```python
from build123d import *

# Parameters (mm, degrees)
BOSS_EXTRU_1_DEPTH      = 3
CONG_1_R                = 5
ESQUISSE2_R             = 1
ENL_V_MAT_EXTRU_1_DEPTH = 257.837010573
D_GAGEMENT_M31_D        = 3.4
ESQUISSE5_R             = 12
ESQUISSE5_R_2           = 11
ESQUISSE5_R_3           = 1.5
ESQUISSE5_R_4           = 1
ESQUISSE5_W             = 50
ESQUISSE5_H             = 10
ENL_V_MAT_EXTRU_2_DEPTH = 257.837010573
D_GAGEMENT_M32_D        = 3.4
D_GAGEMENT_M32_DEPTH    = 3


with BuildPart() as part:
    # Esquisse1 → Boss.-Extru.1 (new body)
    with BuildSketch(Plane(origin=(0, 0, 0), x_dir=(1, 0, 0), z_dir=(0, 1, 0))):
        Polygon((-92.5, 0), (92.5, 0), (132.5, 40), (132.5, 220), (102.5, 220), (85.179491924, 190), (-85.179491924, 190), (-102.5, 220), (-132.5, 220), (-132.5, 40), align=None)
    extrude(amount=BOSS_EXTRU_1_DEPTH)

    # Congé1
    cong_1_edges = [part.edges().sort_by_distance(p)[0] for p in [
        (92.5, 1.5, 0),
        (-92.5, 1.5, 0),
        (-132.5, 1.5, -40),
        (-132.5, 1.5, -220),
        (-102.5, 1.5, -220),
        (-85.179491924, 1.5, -190),
        (85.179491924, 1.5, -190),
        (102.5, 1.5, -220),
        (132.5, 1.5, -220),
        (132.5, 1.5, -40),
    ]]
    fillet(cong_1_edges, radius=CONG_1_R)

    # Esquisse2 → Enlèv. mat.-Extru.1 (cut, through all)
    with BuildSketch(Plane.XZ):
        with Locations(Location((-70, -8, 0), (0, 0, 270))):
            Circle(ESQUISSE2_R)
        with Locations(Location((-124.5, -70, 0), (0, 0, 270))):
            Circle(ESQUISSE2_R)
        with Locations(Location((-124.5, -212, 0), (0, 0, 270))):
            Circle(ESQUISSE2_R)
        with Locations(Location((124.5, -212, 0), (0, 0, 90))):
            Circle(ESQUISSE2_R)
        with Locations(Location((124.5, -70, 0), (0, 0, 90))):
            Circle(ESQUISSE2_R)
        with Locations(Location((70, -8, 0), (0, 0, 90))):
            Circle(ESQUISSE2_R)
    extrude(amount=-ENL_V_MAT_EXTRU_1_DEPTH, mode=Mode.SUBTRACT)

    # Dégagement M31 (through all)
    with Locations(Plane(origin=(0, 0, 0), x_dir=(-1, 0, 0), z_dir=(0, -1, 0))):
        with Locations((-70, 8), (-124.5, 70), (-124.5, 212), (124.5, 212), (124.5, 70), (70, 8)):
            Hole(D_GAGEMENT_M31_D / 2)

    # Esquisse5 → Enlèv. mat.-Extru.2 (cut, through all)
    with BuildSketch(Plane.XZ):
        with Locations(Location((-97.5, -36, 0), (0, 0, 270))):
            Circle(ESQUISSE5_R)
        with Locations(Location((97.5, -55, 0), (0, 0, 270))):
            Circle(ESQUISSE5_R_2)
        with Locations(Location((97.5, -86, 0), (0, 0, 270))):
            Circle(ESQUISSE5_R_3)
        with Locations(Location((97.5, -24, 0), (0, 0, 270))):
            Circle(ESQUISSE5_R_3)
        with Locations(Location((-35, -138, 0), (0, 0, 270))):
            Circle(ESQUISSE5_R_4)
        with Locations(Location((-35, -82, 0), (0, 0, 270))):
            Circle(ESQUISSE5_R_4)
        with Locations(Location((35, -130, 0), (0, 0, 270))):
            Circle(ESQUISSE5_R_4)
        with Locations(Location((35, -90, 0), (0, 0, 270))):
            Circle(ESQUISSE5_R_4)
        with Locations(Location((0, -166, 0), (0, 0, 270))):
            Circle(ESQUISSE5_R_3)
        with Locations(Location((-54.5, -54, 0), (0, 0, 270))):
            Circle(ESQUISSE5_R_3)
        with Locations(Location((54.5, -54, 0), (0, 0, 270))):
            Circle(ESQUISSE5_R_3)
        with Locations(Location((-87.5, -74, 0), (0, 0, 270))):
            Circle(ESQUISSE5_R_3)
        with Locations(Location((-87.5, -165, 0), (0, 0, 270))):
            Circle(ESQUISSE5_R_3)
        with Locations(Location((-32.335, -50, 0), (0, 0, 270))):
            Circle(ESQUISSE5_R_3)
        with Locations(Location((-32.335, -10, 0), (0, 0, 270))):
            Circle(ESQUISSE5_R_3)
        with Locations(Location((32.335, -10, 0), (0, 0, 270))):
            Circle(ESQUISSE5_R_3)
        with Locations(Location((32.335, -50, 0), (0, 0, 270))):
            Circle(ESQUISSE5_R_3)
        with Locations((2.5, -82)):
            Rectangle(ESQUISSE5_W, ESQUISSE5_H)
    extrude(amount=-ENL_V_MAT_EXTRU_2_DEPTH, mode=Mode.SUBTRACT)

    # Dégagement M32
    with Locations(Plane(origin=(0, 3, 0), x_dir=(1, 0, 0), z_dir=(0, 1, 0))):
        with Locations((97.5, 86), (97.5, 24), (-54.5, 54), (54.5, 54), (0, 166), (-87.5, 74), (-87.5, 165), (-32.335, 50), (-32.335, 10), (32.335, 10), (32.335, 50), (-35, 138), (-35, 82), (35, 90), (35, 130)):
            Hole(D_GAGEMENT_M32_D / 2, depth=D_GAGEMENT_M32_DEPTH)


solid = part.part
```
Could you check a few things on this model? Use its own coordinates, in mm. A direction names the side the tool comes from. Give positions to 0.01 mm unless a question says otherwise; leave off trailing zeros. Loops run counter-clockwise (first coordinate to the right, second up) from the corner with the lowest first, then second, coordinate; pieces in that order, holes last. Notation, with made-up numbers: (-30.75, 29) - (7.25, 29) arc R13 ccw to (7.25, 34) - close; hole circle Ø6 at (-18, 20.25). An arc over 180 degrees is marked (long way). Use one line per item in the form item = value.
1. On a 3-axis mill with a long thin cutter (end or side, diameter ignored), from which of +Z, -Z, +X, -X, +Y, -Y can I reach the whole of each face in a straight line? I mean faces 1 (the face through (-2, 3, -112)), 2 (the face through (93.941, 1.479, -205.175)). Say none if no direction works.
Response values:
face_1 = +Z, -Z, +X, -X, +Y
face_2 = -Z, +Y, -Y
2. I want a section at A-A (z = -206). Please give me the cut outline in (x, y), and give its area (3 significant figures).
Response values:
outline = (-132.5, 0) - (-94.42, 0) - (-94.42, 3) - (-132.5, 3) - close; (94.42, 0) - (132.5, 0) - (132.5, 3) - (94.42, 3) - close
area = 228 mm²
3. I'm going to push a flat-ended pin straight in: pin 1 Ø2.5 at (x, z) = (-32.335, -50) entering from -Y. Where does the tip first touch, or does it pass through?
Response values:
pin_1 = through
4. Thinking about a two-plate mould opening in X: for faces 3 (the face through (108.406, 1.479, -53.568)), 4 (the face through (-2, 0, -112)), 5 (the face through (-112.8, 1.5, -20.3)), which applies, released by +X, released by -X, zero draft, split by the parting line, or undercut?
Response values:
face_3 = undercut
face_4 = zero draft
face_5 = released by -X
5. I want a section at B-B (y = 1.35). Give the number of separate pieces and of enclosed holes in the cut face, and give its area (3 significant figures).
Response values:
separate_pieces = 1
enclosed_holes = 24
area = 49,500 mm²
6. I need wall thicknesses on probe 1 along Z at (x, y) = (35, 1.1); probe 2 along Z at (x, y) = (-35, 1.85); probe 3 along X at (y, z) = (0.85, -70). Which ranges of each line are inside material? Lowest first, please.
Response values:
probe_1 = -190 to -131.7, -128.3 to -91.7, -88.3 to 0
probe_2 = -190 to -139.7, -136.3 to -83.7, -80.3 to 0
probe_3 = -132.5 to -126.2, -122.8 to 122.8, 126.2 to 132.5
